Part print with two shaded views. Sizes in mm from the minimum x, y, z corner. Round coordinates to 2 decimals unless told otherwise and drop trailing zeros. Loops run counter-clockwise (first coordinate to the right, second up) from the corner with the lowest first, then second, coordinate; pieces in that order, holes last. Notation, with made-up numbers: M -19,83 L 33,83 A21 cw 33,105 Z; hole C 46,89 d3. An arc over 180 degrees is marked long. Put each result on its own line as item: value. Start each with the question number.
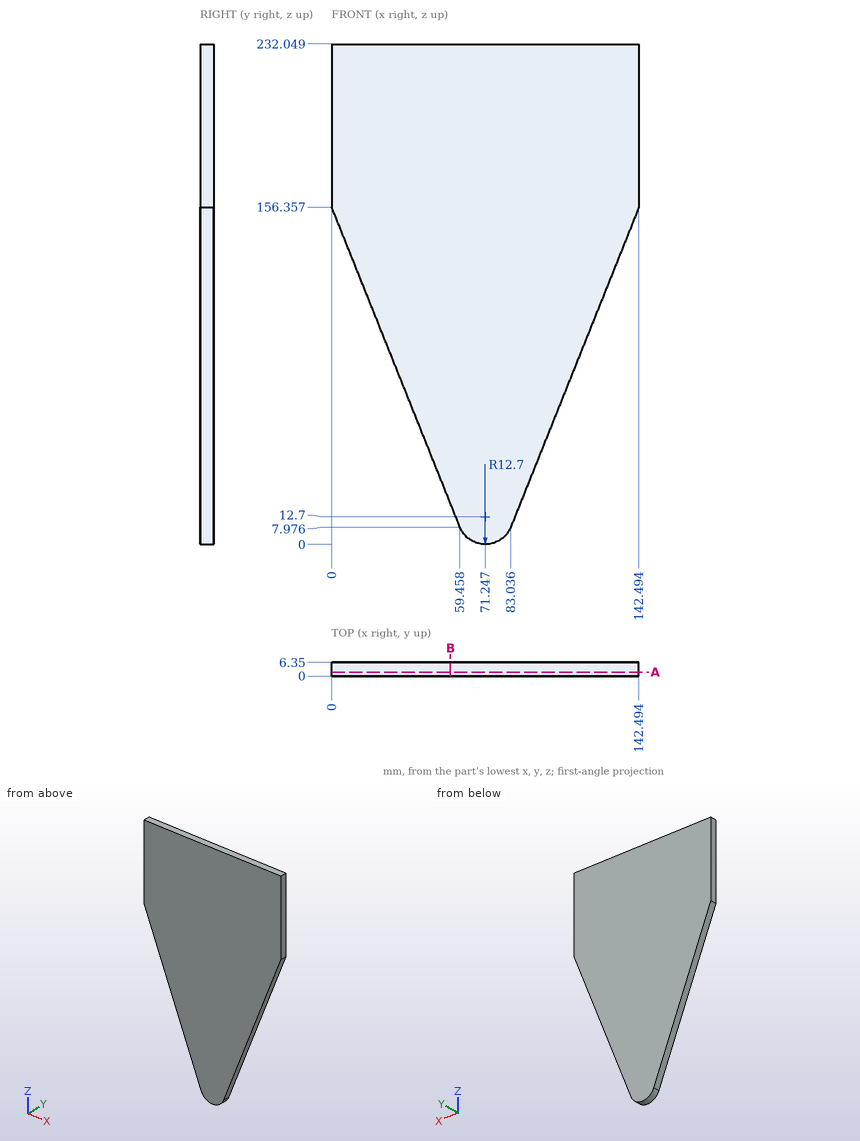
(1) Cut at B-B on x = 55. List the corners of the cut face in (y, z), and give its area (3 significant figures).
(2) Flat gauge pins, fed straight in: pin 1 Ø2 at (x, z) = (60.5, 149.5) entering from -Y; pin 2 Ø1 at (x, y) = (109.5, 2.5) entering from -Z; pin 3 Ø1 at (x, y) = (112.5, 2) entering from -Z. Where does each tip first touch, or does it go through?
(3) Cut at A-A on y = 1.75. List the corners of the cut face in (x, z), and give its area (3 significant figures).
(4) Drill centre lines: line 1 along Z through (x, y) = (72, 4.5); line 2 along X through (y, z) = (0.5, 48); line 3 along X through (y, z) = (4.75, 126) (1 decimal). Where is each one in solid material? Low to high.
Taken from the geometry:
1. outline: M 0,19.1 L 6.35,19.1 L 6.35,232.05 L 0,232.05 Z
1. area: 1,350 mm2
2. pin 1: y = 0
2. pin 2: z = 72.77
2. pin 3: z = 80.26
3. outline: M 0,156.36 L 59.46,7.98 A12.7 ccw 83.04,7.98 L 142.49,156.36 L 142.49,232.05 L 0,232.05 Z
3. area: 23,200 mm2
4. line 1: 0.02 to 232.05
4. line 2: 43.42 to 99.07
4. line 3: 12.2 to 130.3
